Check sheet for the drawn part. Datum: minimum x, y, z corner. Units: mm. A direction names the side the tool comes from. Round coordinates to 2 decimals unless told otherwise and drop trailing zeros. Order: outer loops, then holes, each group sorted by start corner. A loop starts at its lowest first (then second) coordinate and runs counter-clockwise, first axis right, second up. Notation, with made-up numbers: (59, 71) -> (75, 71) arc R7 cw to (75, 75) -> close; hole circle Ø10 at (6.5, 80.5). An arc over 180 degrees is marked (long way). Answer in a Markdown table with one row per item.
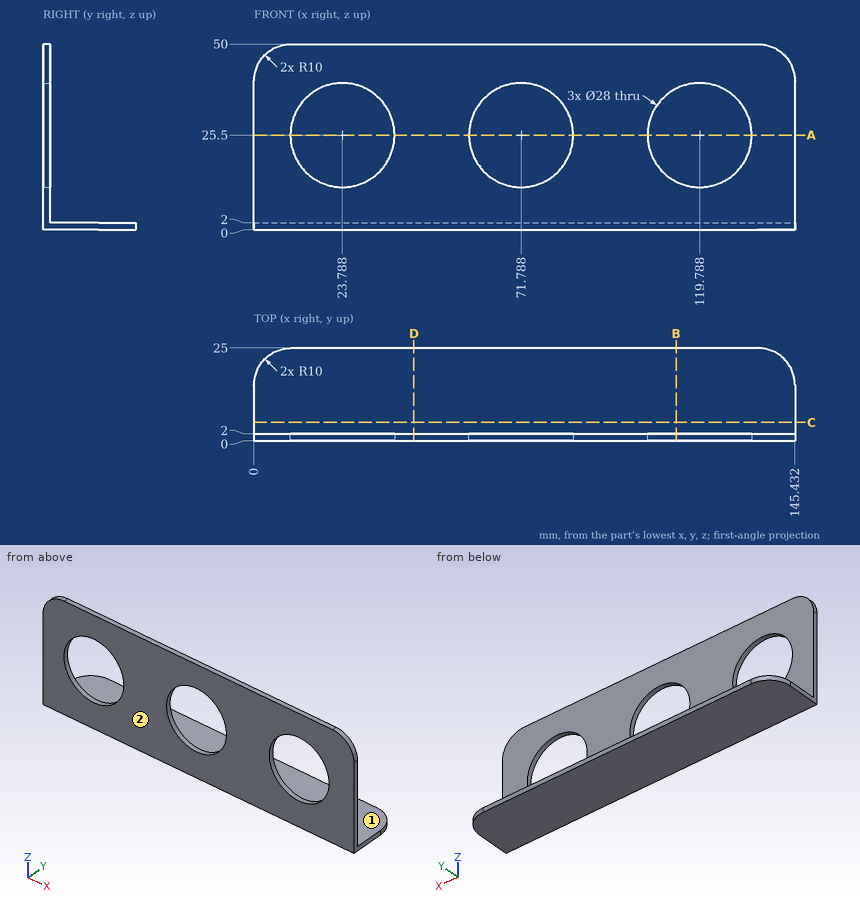
(1) Scan line: probe 1 along Y at (x, z) = (71.5, 6.5). Record every from-to range of solid material in increasing order. Write a range as from..to.
Solutions:
| item | result |
|---|---|
| probe 1 | 0..2 |
(2) Section check B-B on x = 113.5. Record the boundary of the cut face in (y, z).
Solutions:
| item | result |
|---|---|
| outline | (0, 0) -> (25, 0) -> (25, 2) -> (2, 2) -> (2, 12.99) -> (0, 12.99) -> close; (0, 38.01) -> (2, 38.01) -> (2, 50) -> (0, 50) -> close |
(3) Section check C-C on y = 5. Record the boundary of the cut face in (x, z).
Solutions:
| item | result |
|---|---|
| outline | (0, 0) -> (145.43, 0) -> (145.43, 2) -> (0, 2) -> close |
(4) Section check A-A on z = 25.5. Record the boundary of the cut face in (x, y), plus the area to 3 significant figures.
Solutions:
| item | result |
|---|---|
| outline | (0, 0) -> (9.79, 0) -> (9.79, 2) -> (0, 2) -> close; (37.79, 0) -> (57.79, 0) -> (57.79, 2) -> (37.79, 2) -> close; (85.79, 0) -> (105.79, 0) -> (105.79, 2) -> (85.79, 2) -> close; (133.79, 0) -> (145.43, 0) -> (145.43, 2) -> (133.79, 2) -> close |
| area | 123 mm^2 |
(5) Section check D-D on x = 43. Record the boundary of the cut face in (y, z).
Solutions:
| item | result |
|---|---|
| outline | (0, 0) -> (25, 0) -> (25, 2) -> (2, 2) -> (2, 50) -> (0, 50) -> close |
(6) Tool access check on the marked faces 1 and 2. Record the directions out of +Z, -Z, +X, -X, +Y, -Y that give a thin tool (end or side, any length) a straight path to the whole face; none if there is none.
Solutions:
| item | result |
|---|---|
| face 1 | +Z, +X, -X, +Y |
| face 2 | +Z, -Z, +X, -X, -Y |
(7) Depth check by flat-ended pin: pin 1 Ø11.5 at (x, y) = (100, 12.5) entering from +Z; pin 2 Ø1 at (x, z) = (102, 26.5) entering from +Y; pin 3 Ø22.5 at (x, z) = (23.79, 25.5) entering from +Y. Enter the tip coordinate at first touch or a pass-through.
Solutions:
| item | result |
|---|---|
| pin 1 | z = 2 |
| pin 2 | y = 2 |
| pin 3 | through |
